from build123d import *

# Parameters (mm, degrees)
BOSS_EXTRUDE1_DEPTH  = 950
CUT_EXTRUDE1_REACH   = 1533.987
BOSS_EXTRUDE2_REACH  = 1533.987
SKETCH4_W            = 970
SKETCH4_H            = 267.941802888
CUT_EXTRUDE2_DEPTH   = 480
BOSS_EXTRUDE4_DEPTH  = 50
SKETCH14_W           = 25
SKETCH14_H           = 138.177258536
BOSS_EXTRUDE9_DEPTH  = 25
BOSS_EXTRUDE10_START = -25
BOSS_EXTRUDE10_DEPTH = 25
BOSS_EXTRUDE11_DEPTH = 25
BOSS_EXTRUDE12_DEPTH = 25
SKETCH18_W           = 160
SKETCH18_H           = 25
BOSS_EXTRUDE13_DEPTH = 25
SKETCH19_W           = 274.073507304
SKETCH19_H           = 800
CUT_EXTRUDE3_DEPTH   = 25
CUT_EXTRUDE4_DEPTH   = 1168.808883951
CUT_EXTRUDE5_START   = -45
SKETCH22_W           = 788
SKETCH22_H           = 6
CUT_EXTRUDE5_DEPTH   = 350
BOSS_EXTRUDE14_DEPTH = 15
SKETCH24_W           = 650
SKETCH24_H           = 750
BOSS_EXTRUDE15_DEPTH = 15
SKETCH25_W           = 680
SKETCH25_H           = 370
BOSS_EXTRUDE16_DEPTH = 15
CUT_EXTRUDE6_REACH   = 2042.828
SKETCH26_W           = 185
SKETCH26_H           = 185


with BuildPart() as part:
    # Sketch1 → Boss-Extrude1 (new body)
    with BuildSketch(Plane.XY):
        with BuildLine():
            Line((-625, 133.722285201), (-340, -21.277714799))
            Line((-340, -21.277714799), (-340, -271.277714799))
            Line((-340, -271.277714799), (340, -271.277714799))
            Line((340, -271.277714799), (340, -21.277714799))
            Line((340, -21.277714799), (625, 133.722285201))
            ThreePointArc((625, 133.722285201), (589.16333328, 227.263719871), (500, 272.916394272))
            Line((500, 272.916394272), (500, 422.916394272))
            Line((500, 422.916394272), (485, 422.916394272))
            Line((485, 422.916394272), (485, 407.916394272))
            Line((485, 407.916394272), (485, 258.722285201))
            ThreePointArc((485, 258.722285201), (570.238559505, 225.151973889), (609.693359356, 142.472492778))
            Line((609.693359356, 142.472492778), (325, -12.360737749))
            Line((325, -12.360737749), (325, -256.277714799))
            Line((325, -256.277714799), (-325, -256.277714799))
            Line((-325, -256.277714799), (-325, -12.360737749))
            Line((-325, -12.360737749), (-609.693359356, 142.472492778))
            ThreePointArc((-609.693359356, 142.472492778), (-570.238559505, 225.151973889), (-485, 258.722285201))
            Line((-485, 258.722285201), (-485, 407.916394272))
            Line((-485, 407.916394272), (-485, 422.916394272))
            Line((-485, 422.916394272), (-500, 422.916394272))
            Line((-500, 422.916394272), (-500, 272.916394272))
            ThreePointArc((-500, 272.916394272), (-589.16333328, 227.263719871), (-625, 133.722285201))
        make_face()
    extrude(amount=BOSS_EXTRUDE1_DEPTH)

    # Cut-Extrude1: up to this face of the body (flat: up to its plane)
    cut_extrude1_end = Plane(part.part.faces().sort_by_distance((-500, 347.916394272, 475))[0])
    # Sketch2 → Cut-Extrude1 (cut, up to the picked face)
    with BuildSketch(Plane(origin=(500, 0, 0), x_dir=(0, 0, -1), z_dir=(1, 0, 0)), mode=Mode.PRIVATE) as cut_extrude1_sk1:
        Polygon((-950, 358.722285201), (0, 422.916394272), (-950, 422.916394272), align=None)
    cut_extrude1_tool1 = split(extrude(cut_extrude1_sk1.sketch, amount=-CUT_EXTRUDE1_REACH, mode=Mode.PRIVATE), bisect_by=cut_extrude1_end, keep=Keep.BOTH, mode=Mode.PRIVATE)
    add(cut_extrude1_tool1.solids().sort_by(Axis((500, 401.518358, 633.333333), (-1, 0, 0)))[0], mode=Mode.SUBTRACT)

    # Boss-Extrude2: up to this face of the body (flat: up to its plane)
    boss_extrude2_end = Plane(part.part.faces().sort_by_distance((500, 333.324179095, 431.896465862))[0])
    # Sketch3 → Boss-Extrude2 (add, up to the picked face)
    with BuildSketch(Plane.ZY.offset(500), mode=Mode.PRIVATE) as boss_extrude2_sk1:
        Polygon((800, 368.85819716), (890, 540.85819716), (1030, 497.85819716), (1280, 459.85819716), (1280, 272.916394272), (800, 272.916394272), align=None)
    boss_extrude2_tool1 = split(extrude(boss_extrude2_sk1.sketch, amount=-BOSS_EXTRUDE2_REACH, mode=Mode.PRIVATE), bisect_by=boss_extrude2_end, keep=Keep.BOTH, mode=Mode.PRIVATE)
    add(boss_extrude2_tool1.solids().sort_by(Axis((-500, 382.129187, 1038.198063), (1, 0, 0)))[0])

    # Sketch4 → Cut-Extrude2 (cut)
    with BuildSketch(Plane.XY.offset(1280)):
        with Locations((0, 406.887295716)):
            Rectangle(SKETCH4_W, SKETCH4_H)
    extrude(amount=-CUT_EXTRUDE2_DEPTH, mode=Mode.SUBTRACT)

    # Sketch9 → Boss-Extrude4 (add)
    with BuildSketch(Plane.XY.offset(950)):
        Polygon((-609.693359356, 142.472492778), (-616.859938559, 129.295234242), (-340, -21.277714799), (-332.833420796, -8.100456263), align=None)
    boss_extrude4 = extrude(amount=BOSS_EXTRUDE4_DEPTH)

    # Sketch14 → Boss-Extrude9 (add)
    with BuildSketch(Plane(origin=(-485, 0, 0), x_dir=(0, 0, -1), z_dir=(1, 0, 0))):
        with Locations((-862.5, 327.810914469)):
            Rectangle(SKETCH14_W, SKETCH14_H)
    boss_extrude9 = extrude(amount=BOSS_EXTRUDE9_DEPTH)

    # Sketch15 → Boss-Extrude10 (add)
    with BuildSketch(Plane.XY.offset(875).offset(BOSS_EXTRUDE10_START)):
        with BuildLine():
            Line((-460, 258.722285201), (-460, 233.722285201))
            Line((-460, 233.722285201), (-485, 233.722285201))
            ThreePointArc((-485, 233.722285201), (-555.050087415, 205.087439536), (-584.98270599, 135.581990265))
            Line((-584.98270599, 135.581990265), (-587.731261796, 130.528194105))
            Line((-587.731261796, 130.528194105), (-609.693359356, 142.472492778))
            ThreePointArc((-609.693359356, 142.472492778), (-570.238559505, 225.151973889), (-485, 258.722285201))
            Line((-485, 258.722285201), (-460, 258.722285201))
        make_face()
    boss_extrude10 = extrude(amount=BOSS_EXTRUDE10_DEPTH)

    # Sketch16 → Boss-Extrude11 (add)
    with BuildSketch(Plane.XY.offset(875)):
        Polygon((-587.731261796, 130.528194105), (-325, -12.360737749), (-325, 12.639262251), (-583.120237767, 153.020444195), align=None)
    boss_extrude11 = extrude(amount=-BOSS_EXTRUDE11_DEPTH)

    # Sketch17 → Boss-Extrude12 (add)
    with BuildSketch(Plane.XY.offset(875)):
        Polygon((-325, 12.639262251), (-325, 392.639262251), (-350, 392.639262251), (-350, 26.23575348), align=None)
    boss_extrude12 = extrude(amount=-BOSS_EXTRUDE12_DEPTH)

    # Sketch18 → Boss-Extrude13 (add)
    with BuildSketch(Plane.XY.offset(875)):
        with Locations((-405, 405.139262251)):
            Rectangle(SKETCH18_W, SKETCH18_H)
    boss_extrude13 = extrude(amount=-BOSS_EXTRUDE13_DEPTH)

    # Sketch19 → Cut-Extrude3 (cut)
    with BuildSketch(Plane(origin=(-79.374447411, -145.946564595, 0), x_dir=(0.8784839023828743, -0.47777194690998404, 0), z_dir=(0.47777194690998404, 0.8784839023828743, 0))):
        with Locations((-441.638408187, -425)):
            Rectangle(SKETCH19_W, SKETCH19_H)
    cut_extrude3 = extrude(amount=-CUT_EXTRUDE3_DEPTH, mode=Mode.SUBTRACT)

    # Sketch21 → Cut-Extrude4 (cut, symmetric)
    with BuildSketch(Plane(origin=(0, 0, 825), x_dir=(-1, 0, 0), z_dir=(0, 0, -1))):
        Polygon((584.610332143, 123.708384863), (354.382974735, -1.502984955), (357.249606416, -6.773888369), (587.476963824, 118.437481449), align=None)
    cut_extrude4 = extrude(amount=CUT_EXTRUDE4_DEPTH, both=True, mode=Mode.SUBTRACT)

    # Sketch22 → Cut-Extrude5 (cut)
    with BuildSketch(Plane(origin=(-508.356814385, 276.4747587, 0), x_dir=(0, 0, -1), z_dir=(0.8784839023828743, -0.477771946909984, 0)).offset(CUT_EXTRUDE5_START)):
        with Locations((-425, -173.634591879)):
            Rectangle(SKETCH22_W, SKETCH22_H)
    cut_extrude5 = extrude(amount=CUT_EXTRUDE5_DEPTH, mode=Mode.SUBTRACT)

    # Mirror1: Boss-Extrude4, Boss-Extrude9, Boss-Extrude10, Boss-Extrude11, Boss-Extrude12, Boss-Extrude13, Cut-Extrude3, Cut-Extrude4, Cut-Extrude5 across plane
    add(boss_extrude4.mirror(Plane(origin=(0, 0, 0), x_dir=(0, 0, 1), z_dir=(1, 0, 0))))
    add(boss_extrude9.mirror(Plane(origin=(0, 0, 0), x_dir=(0, 0, 1), z_dir=(1, 0, 0))))
    add(boss_extrude10.mirror(Plane(origin=(0, 0, 0), x_dir=(0, 0, 1), z_dir=(1, 0, 0))))
    add(boss_extrude11.mirror(Plane(origin=(0, 0, 0), x_dir=(0, 0, 1), z_dir=(1, 0, 0))))
    add(boss_extrude12.mirror(Plane(origin=(0, 0, 0), x_dir=(0, 0, 1), z_dir=(1, 0, 0))))
    add(boss_extrude13.mirror(Plane(origin=(0, 0, 0), x_dir=(0, 0, 1), z_dir=(1, 0, 0))))
    add(cut_extrude3.mirror(Plane(origin=(0, 0, 0), x_dir=(0, 0, 1), z_dir=(1, 0, 0))), mode=Mode.SUBTRACT)
    add(cut_extrude4.mirror(Plane(origin=(0, 0, 0), x_dir=(0, 0, 1), z_dir=(1, 0, 0))), mode=Mode.SUBTRACT)
    add(cut_extrude5.mirror(Plane(origin=(0, 0, 0), x_dir=(0, 0, 1), z_dir=(1, 0, 0))), mode=Mode.SUBTRACT)

    # Sketch23 → Boss-Extrude14 (add)
    with BuildSketch(Plane.ZY.offset(340)):
        Polygon((950, -271.277714799), (1700, -271.277714799), (1700, 98.722285201), (950, 208.722285201), (873.5, 208.722285201), (873.5, -21.277714799), (950, -21.277714799), align=None)
    boss_extrude14 = extrude(amount=-BOSS_EXTRUDE14_DEPTH)

    # Mirror2: Boss-Extrude14 across plane
    add(boss_extrude14.mirror(Plane(origin=(0, 0, 0), x_dir=(0, 0, 1), z_dir=(1, 0, 0))))

    # Sketch24 → Boss-Extrude15 (add)
    with BuildSketch(Plane(origin=(0, -256.277714799, 0), x_dir=(1, 0, 0), z_dir=(0, 1, 0))):
        with Locations((0, -1325)):
            Rectangle(SKETCH24_W, SKETCH24_H)
    extrude(amount=-BOSS_EXTRUDE15_DEPTH)

    # Sketch25 → Boss-Extrude16 (add)
    with BuildSketch(Plane.XY.offset(1700)):
        with Locations((0, -86.277714799)):
            Rectangle(SKETCH25_W, SKETCH25_H)
    extrude(amount=BOSS_EXTRUDE16_DEPTH)

    # Cut-Extrude6: up to this face of the body (flat: up to its plane)
    cut_extrude6_end = Plane(part.part.faces().sort_by_distance((-340, -90.018652178, 958.920592754))[0])
    # Sketch26 → Cut-Extrude6 (cut, up to the picked face)
    with BuildSketch(Plane(origin=(340, 0, 0), x_dir=(0, 0, -1), z_dir=(1, 0, 0)), mode=Mode.PRIVATE) as cut_extrude6_sk1:
        with Locations((-1152.5, 26.222285201)):
            Rectangle(SKETCH26_W, SKETCH26_H)
    cut_extrude6_tool1 = split(extrude(cut_extrude6_sk1.sketch, amount=-CUT_EXTRUDE6_REACH, mode=Mode.PRIVATE), bisect_by=cut_extrude6_end, keep=Keep.BOTH, mode=Mode.PRIVATE)
    add(cut_extrude6_tool1.solids().sort_by(Axis((340, 26.222285, 1152.5), (-1, 0, 0)))[0], mode=Mode.SUBTRACT)


solid = part.part
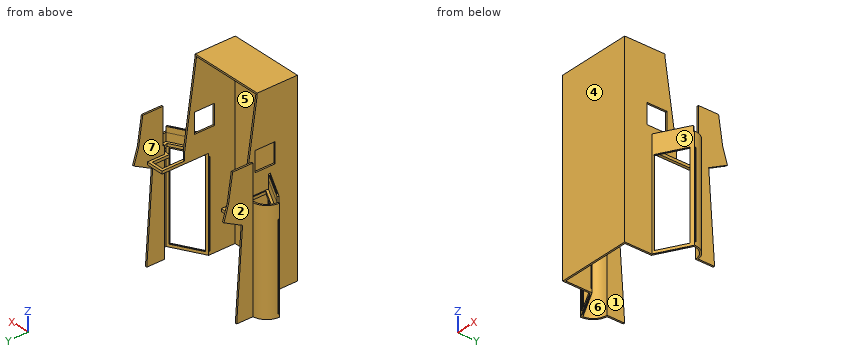
Build history of the part. All positions in model axes, mm. Face numbers are marked on the shaded views. A direction names the side the tool comes from. Round coordinates to 2 decimals unless told otherwise and drop trailing zeros. Write each loop counter-clockwise with the first axis right and the second up, starting at its lowest first coordinate (ties: lowest second). Pieces come first, ordered by that corner, then holes. Notation, with made-up numbers: (25, 75.25) - (70, 75.25) arc R22 cw to (70, 103.25) - close; hole circle Ø1 at (85.25, 62.5). An arc over 180 degrees is marked (long way). Use CSV: the item, a comma, the result in double quotes.
(1) Band-saw the part on A-A (x = 420). Write the cut outline in (y, z), plus the area to 3 significant figures.
Response:
outline,"(22.23, 0) - (27.35, 0) - (27.35, 25) - (22.23, 25) - close; (22.23, 825) - (27.35, 825) - (27.35, 1000) - (22.23, 1000) - close; (34.18, 0) - (39.31, 0) - (39.31, 25) - (34.18, 25) - close; (34.18, 825) - (39.31, 825) - (39.31, 850) - (64.31, 850) - (64.31, 875) - (39.31, 875) - (39.31, 1000) - (34.18, 1000) - close; (392.64, 850) - (417.64, 850) - (417.64, 875) - (392.64, 875) - close"
area,"3,300 mm²"
(2) Band-saw the part on C-C (z = 1477.5). Write the cut outline in (x, y).
Response:
outline,"(-340, -271.28) - (340, -271.28) - (340, 131.36) - (325, 131.36) - (325, -256.28) - (-325, -256.28) - (-325, 131.36) - (-340, 131.36) - close"
(3) Wall check: line 1 (X direction, y = 171, z = 954.5); line 2 (X direction, y = 242.5, z = 866); line 3 (Y direction, x = 301, z = 391). Give the ranges that are in metal, low to high.
Response:
line 1,"-340 to -325, 325 to 340"
line 2,"-573.13 to -460, -350 to -325, 325 to 350, 460 to 573.13"
line 3,"-271.28 to -256.28"
(4) 3-axis set-ups, long thin cutter, end or side, ignore diameter. For the marked faces 5, 6 and 7: which of +Z, -Z, +X, -X, +Y, -Y reach the whole face in a straight line?
Response:
face 5,"-Z, +Y"
face 6,"-Z"
face 7,"+Y"
(5) Band-saw the part on D-D (x = 191.5). Write the cut outline in (y, z).
Response:
outline,"(-271.28, 0) - (-256.28, 0) - (-256.28, 1700) - (98.72, 1700) - (98.72, 1715) - (-271.28, 1715) - close"
(6) Band-saw the part on B-B (y = -153). Write the cut outline in (x, z).
Response:
outline,"(-340, 0) - (-325, 0) - (-325, 1700) - (325, 1700) - (325, 0) - (340, 0) - (340, 1715) - (-340, 1715) - close"
(7) Mould opens along X. For the marked faces 1, 2, 3 and 4 say: pulls with the +X half, pulls with the -X half, needs draft (parallel to the pull), parting line crosses it, or undercut.
Response:
face 1,"undercut"
face 2,"pulls with the -X half"
face 3,"pulls with the +X half"
face 4,"needs draft"
(8) Pin check, flat tips, straight feed: P1, Ø16.5, axis at x = 335.5, z = 1137, coming from the +Y side; P2, Ø20, axis at y = 297.5, z = 860.5, coming from the +X side; P3, Ø3, axis at x = -45, z = 1193.5, coming from the +Y side. Stop position of each tip, or through.
Response:
P1,"y = 182.51"
P2,"x = 500"
P3,"y = -256.28"
